```python
from build123d import *

# Parameters (mm, degrees)
F_01_START                = -3
S01_HEAD_R                = 2.75
F_01_HEAD_DEPTH           = 3
S02_NOMINAL_SHANK_R       = 1.5
F_02_NOMINAL_SHANK_DEPTH  = 42
F_03_START                = -3.1
F_03_HEX_KEY_SOCKET_DEPTH = 1.75


with BuildPart() as part:
    # S01 - Head → 01 - Head (new body)
    with BuildSketch(Plane.XY.offset(F_01_START)):
        Circle(S01_HEAD_R)
    extrude(amount=F_01_HEAD_DEPTH)

    # S02 - Nominal shank → 02 - Nominal shank (add)
    with BuildSketch(Plane.XY):
        with Locations(Location((0, 0, 0), (0, 0, 180))):
            Circle(S02_NOMINAL_SHANK_R)
    extrude(amount=F_02_NOMINAL_SHANK_DEPTH)

    # S03 - Hex key socket → 03 - Hex key socket (cut)
    with BuildSketch(Plane.XY.offset(F_03_START)):
        Polygon((1.443375673, 0), (0.721687836, 1.25), (-0.721687836, 1.25), (-1.443375673, 0), (-0.721687836, -1.25), (0.721687836, -1.25), align=None)
    extrude(amount=F_03_HEX_KEY_SOCKET_DEPTH, mode=Mode.SUBTRACT)


solid = part.part
```
The listing builds one solid part. Answer for the finished solid, in the listing's coordinates (mm). A direction names the side the tool comes from. Coordinates: 2 decimals unless noted, no trailing zeros. Order: outer loops, then holes, each group sorted by start corner. A loop starts at its lowest first (then second) coordinate and runs counter-clockwise, first axis right, second up. Notation, with made-up numbers: M 44.5,31 L 86.5,31 A22 cw 86.5,67 Z; hole C -33,-3.5 d6. An arc over 180 degrees is marked long. Answer as a JSON object with one key per item and string values. Group by question number.
1. A tool of negligible diameter and unlimited length cuts with its end or side. For faces 1 (the flat face through (-1.3, -0.6, -3)), 2 (the flat face through (0, -1.25, -2)), 3 (the cylindrical face through (-1.43, -0.45, 20.71)), from which of +Z, -Z, +X, -X, +Y, -Y can it reach the whole face along a straight path? Write none if from no direction.
2. Section D-D on x = 2.35 is taken. Write down the section's boundary in (y, z).
3. Section C-C on z = 28 is taken. Write down the section's boundary in (x, y).
4. Flat-ended cylindrical pins translate along their axes: P1, Ø1, axis at x = -0.5, z = 15, coming from the +Y side; P2, Ø1.5, axis at y = 2, z = 24, coming from the -X side; P3, Ø1, axis at y = 0, z = 13, coming from the -X side. Find the tip coordinate at first contact, or state that the pin passes through.
5. Straight lines are drawn through the part: line 1 (Z direction, x = 1, y = 1.9); line 2 (Y direction, x = 0.1, z = 9.5). For each, find the intervals that lie inside material, in ascending order.
6. Section B-B on y = -0.75 is taken. Write down the section's boundary in (x, z), then the cut area to 3 significant figures.
7. Section A-A on x = 0 is taken. Write down the section's boundary in (y, z).
8. Determine the mould class of faces 4 (the flat face through (1.2, -1.2, 0)), 5 (the flat face through (-1.088, -0.616, -2.187)), 6 (the cylindrical face through (-0.596, -2.685, -1.521)), 7 (the flat face through (-1.08, 0.63, -2.19)) for opening direction Y: released by +Y, released by -Y, zero draft, split by the parting line, or undercut.
Values follow:
{
 "1": {"face 1": "-Z, +X, -X, +Y, -Y", "face 2": "-Z", "face 3": "+Z"},
 "2": {"outline": "M -1.43,-3 L 1.43,-3 L 1.43,0 L -1.43,0 Z"},
 "3": {"outline": "C 0,0 d3"},
 "4": {"P1": "y = 1.5", "P2": "x = -0.83", "P3": "x = -1.5"},
 "5": {"line 1": "-3 to 0", "line 2": "-1.5 to 1.5"},
 "6": {"outline": "M -2.65,-3 L -1.01,-3 L -1.01,-1.35 L 1.01,-1.35 L 1.01,-3 L 2.65,-3 L 2.65,0 L 1.3,0 L 1.3,42 L -1.3,42 L -1.3,0 L -2.65,0 Z", "area": "122 mm2"},
 "7": {"outline": "M -2.75,-3 L -1.25,-3 L -1.25,-1.35 L 1.25,-1.35 L 1.25,-3 L 2.75,-3 L 2.75,0 L 1.5,0 L 1.5,42 L -1.5,42 L -1.5,0 L -2.75,0 Z"},
 "8": {"face 4": "zero draft", "face 5": "undercut", "face 6": "split by the parting line", "face 7": "undercut"}
}
